```python
from build123d import *

# Parameters (mm, degrees)
PAD_DEPTH       = 28
POCKET_DEPTH    = 100
SKETCH002_R     = 1.5
POCKET001_DEPTH = 7
POCKET002_DEPTH = 40
SKETCH004_R     = 1.5
POCKET003_DEPTH = 10
CHAMFER_SIZE    = 1


with BuildPart() as part:
    # Sketch → Pad (new body)
    with BuildSketch(Plane.XZ):
        with BuildLine():
            Line((0, 0), (-54.04, 0))
            ThreePointArc((-54.04, 0), (-57.54, -3.5), (-54.04, -7))
            Line((-54.04, -7), (2.5, -7))
            Line((2.5, -7), (2.5, 15))
            Line((2.5, 15), (20.5, 15))
            Line((20.5, -13), (20.5, 15))
            Line((-51.54, -13), (20.5, -13))
            ThreePointArc((-51.54, 6), (-61.04, -3.5), (-51.54, -13))
            Line((0, 6), (-51.54, 6))
            Line((0, 0), (0, 6))
        make_face()
    extrude(amount=PAD_DEPTH)

    # Sketch001 (on Face10 of Pad) → Pocket (cut)
    with BuildSketch(Plane(origin=(0, 0, 0), x_dir=(0, 0, 1), z_dir=(1, 0, 0))):
        Polygon((1, 28), (6, 23), (6, 28), align=None)
        Polygon((6, 5), (1, 0), (6, 0), align=None)
    extrude(amount=-POCKET_DEPTH, mode=Mode.SUBTRACT)

    # Sketch002 (on Face7 of Pocket) → Pocket001 (cut)
    with BuildSketch(Plane(origin=(0, 0, 6), x_dir=(-1, 0, 0), z_dir=(0, 0, 1))):
        with Locations((27, 14)):
            Circle(SKETCH002_R)
    extrude(amount=-POCKET001_DEPTH, mode=Mode.SUBTRACT)

    # Sketch003 (on Face13 of Pocket001) → Pocket002 (cut)
    with BuildSketch(Plane(origin=(0, 0, 15), x_dir=(-1, 0, 0), z_dir=(0, 0, 1))):
        with BuildLine():
            ThreePointArc((-6.333333, 16.763854), (-15.5, 14), (-6.333333, 11.236146))
            Line((-6.333333, 11.236146), (-4.5, 14))
            Line((-4.5, 14), (-6.333333, 16.763854))
        make_face()
    extrude(amount=-POCKET002_DEPTH, mode=Mode.SUBTRACT)

    # Sketch004 (on Face12 of Pocket002) → Pocket003 (cut)
    with BuildSketch(Plane(origin=(20.5, 0, 0), x_dir=(0, 0, 1), z_dir=(1, 0, 0))):
        with Locations((0, 14)):
            Circle(SKETCH004_R)
    extrude(amount=-POCKET003_DEPTH, mode=Mode.SUBTRACT)

    # Chamfer
    chamfer_edges = [part.edges().sort_by_distance(p)[0] for p in [
        (-59.694753, -28, -8.373397),
        (-15.52, -28, -13),
        (20.5, -28, 1),
        (20.5, -14, -13),
        (20.5, 0, 1),
        (20.5, -14, 15),
        (11.5, 0, 15),
        (11.5, -28, 15),
        (2.5, -14, 15),
        (-15.52, 0, -13),
        (-59.694753, 0, -8.373397),
    ]]
    chamfer(chamfer_edges, length=CHAMFER_SIZE)


solid = part.part
```
For this review, take the finished solid that the model builds, in its own axes (mm). A direction names the side the tool comes from. Coordinates: 2 decimals unless noted, no trailing zeros. Write each loop counter-clockwise with the first axis right and the second up, starting at its lowest first coordinate (ties: lowest second). Pieces come first, ordered by that corner, then holes.
(1) Add section B-B on z = -3.5. Give the boundary of the cut face in (x, y).
(2) Tool access review of faces 1 (the face through (-25, -14, 6)), 2 (the face through (-26, -14, -7)), 3 (the face through (0, -14, 3)), 4 (the face through (5.43, -12.6, 1.2)): name each direction out of +Z, -Z, +X, -X, +Y, -Y from which nothing blocks a thin tool from reaching the whole face with its end or side.
(3) Wall thickness on probe 1 along Y at (x, z) = (10.5, 1.75); probe 2 along X at (y, z) = (-14, 4.1); probe 3 along X at (y, z) = (-10.75, 5): over which ranges is each line inside the solid? List them lowest first.
(4) The part is to be moulded in two halves that separate along X. For faces 5 (the face through (-2, -28, -7.5)), 6 (the face through (14.808, -11.463, 1.196)), 7 (the face through (20.5, -11, 1)), 8 (the face through (-59.307, -27.826, -7.361)), say which applies: +X half, -X half, draft (parallel to the pull), parting line (faces both ways), or undercut.
(5) Add section C-C on y = -20.5. Give the boundary of the cut face in (x, z), then the cut area to 3 significant figures.
(6) Add section D-D on z = 11.5. Give the boundary of the cut face in (x, y).
(7) For pin 1 Ø1 at (x, z) = (-13.5, 5.5) entering from +Y; pin 2 Ø2 at (y, z) = (-6.5, -8) entering from -X; pin 3 Ø1.8 at (y, z) = (-14, 0) entering from -X; pin 4 Ø11.5 at (x, y) = (10.5, -14) entering from +Z, all flat-tipped, find the tip position at first contact; note any pin that passes through.
(8) Add section A-A on x = 10.5. Give the boundary of the cut face in (y, z).
Answer sheet:
1. outline: (-61.04, -27) - (-60.04, -28) - (-57.54, -28) - (-57.54, 0) - (-60.04, 0) - (-61.04, -1) - close; (2.5, -28) - (19.5, -28) - (20.5, -27) - (20.5, -1) - (19.5, 0) - (2.5, 0) - close; hole (4.5, -14) - (6.33, -16.76) arc R5 ccw (long way) to (6.33, -11.24) - close
2. face 1: +Z, -X, +Y, -Y
2. face 2: +Y, -Y
2. face 3: +Z, +Y, -Y
2. face 4: +Z, -Z
3. probe 1: y = -28 to -19, -9 to 0
3. probe 2: x = -57.24 to -28.5, -25.5 to 0, 2.5 to 4.5, 15.5 to 20.5
3. probe 3: x = -55.78 to 0, 2.5 to 6.7, 14.3 to 20.5
4. face 5: draft
4. face 6: undercut
4. face 7: +X half
4. face 8: -X half
5. outline: (-54.04, -7) arc R3.5 cw to (-54.04, 0) - (0, 0) - (0, 6) - (-51.54, 6) arc R9.5 ccw to (-51.54, -13) - (19.5, -13) - (20.5, -12) - (20.5, 14) - (19.5, 15) - (3.5, 15) - (2.5, 14) - (2.5, -7) - close
5. area: 1,240 mm2
6. outline: (2.5, -28) - (19.5, -28) - (20.5, -27) - (20.5, -1) - (19.5, 0) - (2.5, 0) - close; hole (4.5, -14) - (6.33, -16.76) arc R5 ccw (long way) to (6.33, -11.24) - close
7. pin 1: stops at y = -4
7. pin 2: stops at x = -60.37
7. pin 3: stops at x = -60.68
7. pin 4: stops at z = 15
8. outline: (-28, -12) - (-27, -13) - (-19, -13) - (-19, 15) - (-27, 15) - (-28, 14) - close; (-9, -13) - (-1, -13) - (0, -12) - (0, 14) - (-1, 15) - (-9, 15) - close
